Design review of the part shown in the three views and the two pictorial views. Dimensions are in mm from the part's minimum x, y and z. Coordinates: 2 decimals unless noted, no trailing zeros. Order: outer loops, then holes, each group sorted by start corner. A loop starts at its lowest first (then second) coordinate and runs counter-clockwise, first axis right, second up. Notation, with made-up numbers: (12, -28) - (50, -28) arc R17 ccw to (50, -21) - close; hole circle Ø2 at (71.5, 52). An arc over 180 degrees is marked (long way). One line per item, written item: value. Start each with the question number.
(1) Consider section D-D on x = 12.75. Write out the cut boundary in (y, z), then the cut area to 3 significant figures.
(2) Clearance check with flat-ended pins moving along their axes: pin 1 (1.5 mm diameter, centred on x = 12.5, y = 3, fed in from +Z); pin 2 (3 mm diameter, centred on y = 0.5, z = 12.5, fed in from -X); pin 3 (1.5 mm diameter, centred on x = 14.5, y = 4.5, fed in from -Z). State where each tip first meets the part, or that it passes through.
(3) To check wall thickness, follow line 1 along X through (y, z) = (1.5, 10); line 2 along Z through (x, y) = (5.5, 1.75); line 3 along X through (y, z) = (2.4, 18.25). State the ranges of each line that lie inside material, in increasing order.
(4) Consider section C-C on y = 1.25. Write out the cut boundary in (x, z).
(5) Consider section B-B on z = 10. Write out the cut boundary in (x, y), then the cut area to 3 significant figures.
(6) Consider section A-A on x = 10. Write out the cut boundary in (y, z), then the cut area to 3 significant figures.
(7) Mouldability with a two-part tool opening along Z and no side actions: class the marked faces 1, 2 and 3 as released by +Z, released by -Z, zero draft, split by the parting line, or undercut.
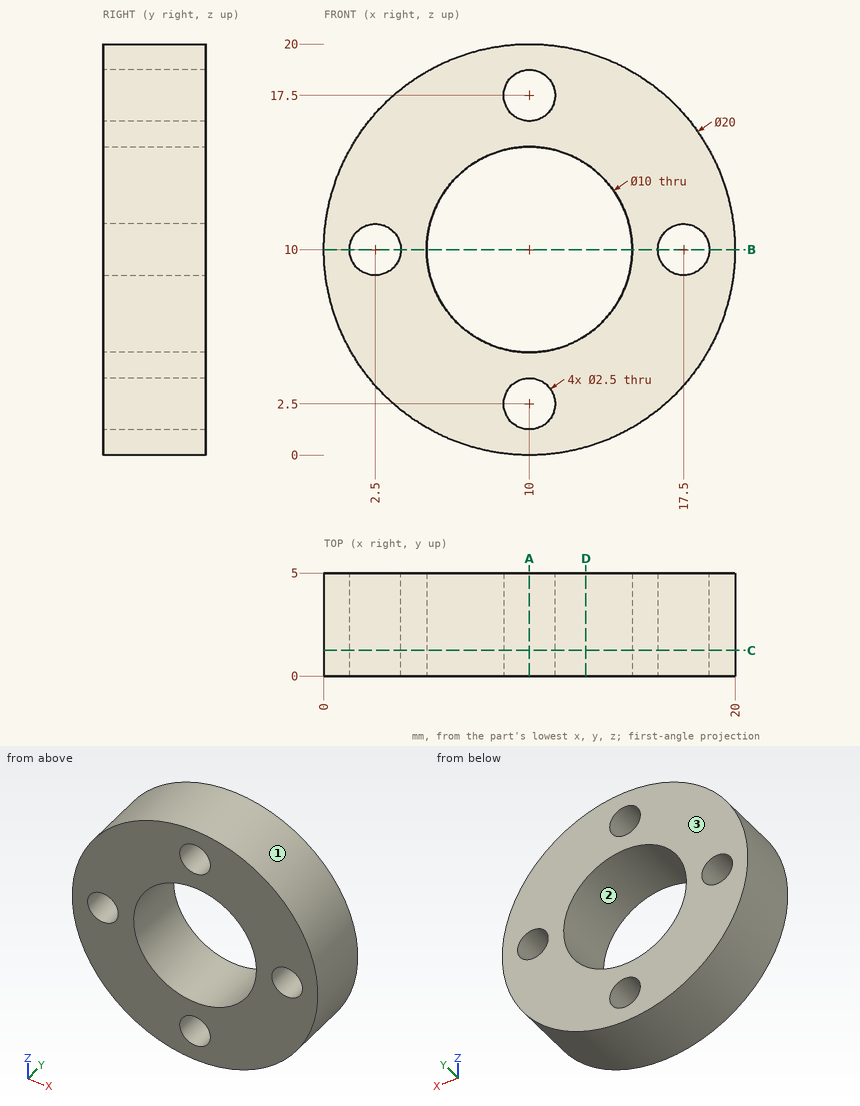
Geometry check:
1. outline: (0, 0.39) - (5, 0.39) - (5, 5.82) - (0, 5.82) - close; (0, 14.18) - (5, 14.18) - (5, 19.61) - (0, 19.61) - close
1. area: 54.4 mm^2
2. pin 1: stops at z = 19.85
2. pin 2: stops at x = 0.05
2. pin 3: stops at z = 0.73
3. line 1: x = 0 to 1.25, 3.75 to 5, 15 to 16.25, 18.75 to 20
3. line 2: z = 1.07 to 7.82, 12.18 to 18.93
3. line 3: x = 4.35 to 9, 11 to 15.65
4. outline: circle Ø20 at (10, 10); hole circle Ø2.5 at (2.5, 10); hole circle Ø10 at (10, 10); hole circle Ø2.5 at (10, 2.5); hole circle Ø2.5 at (10, 17.5); hole circle Ø2.5 at (17.5, 10)
5. outline: (0, 0) - (1.25, 0) - (1.25, 5) - (0, 5) - close; (3.75, 0) - (5, 0) - (5, 5) - (3.75, 5) - close; (15, 0) - (16.25, 0) - (16.25, 5) - (15, 5) - close; (18.75, 0) - (20, 0) - (20, 5) - (18.75, 5) - close
5. area: 25.0 mm^2
6. outline: (0, 0) - (5, 0) - (5, 1.25) - (0, 1.25) - close; (0, 3.75) - (5, 3.75) - (5, 5) - (0, 5) - close; (0, 15) - (5, 15) - (5, 16.25) - (0, 16.25) - close; (0, 18.75) - (5, 18.75) - (5, 20) - (0, 20) - close
6. area: 25.0 mm^2
7. face 1: split by the parting line
7. face 2: undercut
7. face 3: zero draft
